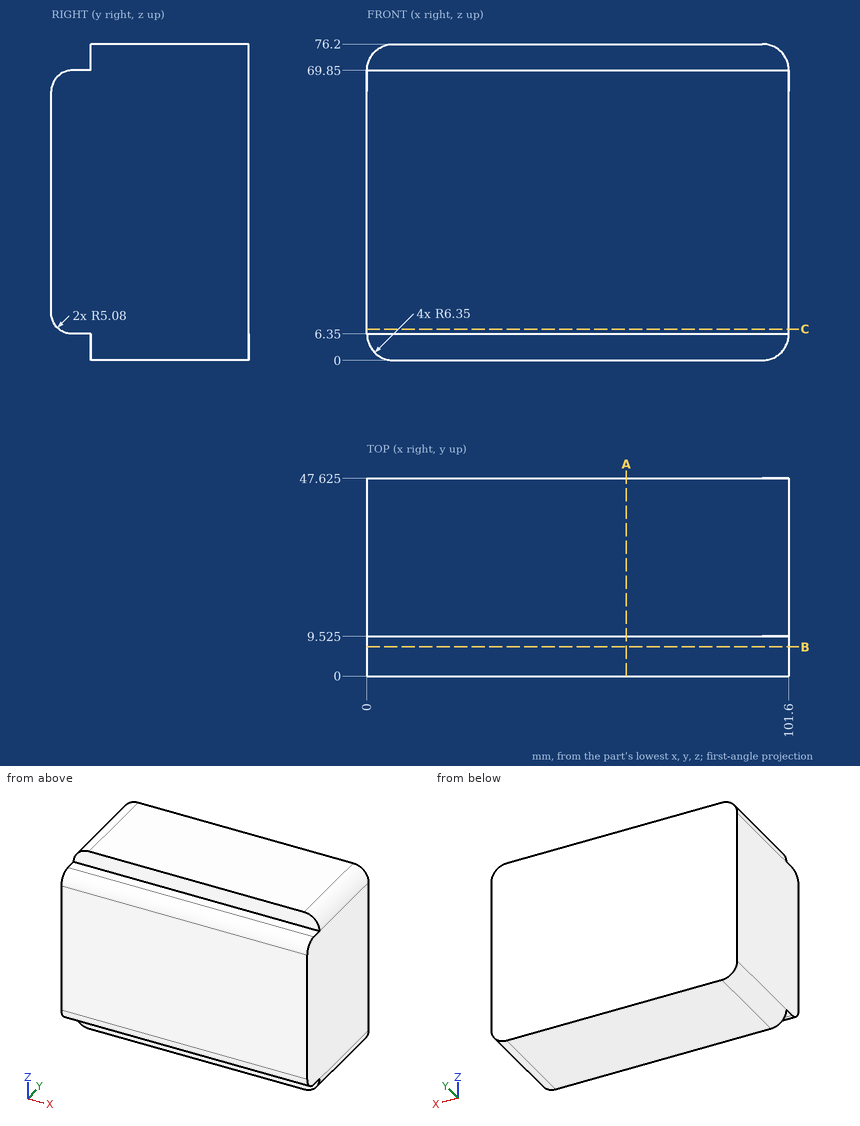
Geometry: see drawing. Coordinates: mm, zero at the bounding-box minimum. Round coordinates to 2 decimals unless told otherwise and drop trailing zeros. Loops run counter-clockwise (first coordinate to the right, second up) from the corner with the lowest first, then second, coordinate; pieces in that order, holes last. Notation, with made-up numbers: (84.25, 87.5) -> (125.25, 87.5) arc R28 cw to (125.25, 111.5) -> close; hole circle Ø10 at (-38, 24). An arc over 180 degrees is marked (long way). Write each question's results on one line, items separated by ' | '.
1. Section A-A (x = 62.5). Return loops of the section in (y, z) (3 decimals).
Geometry results:
outline: (0, 11.43) arc R5.08 ccw to (5.08, 6.35) -> (9.525, 6.35) -> (9.525, 0) -> (47.625, 0) -> (47.625, 76.2) -> (9.525, 76.2) -> (9.525, 69.85) -> (5.08, 69.85) arc R5.08 ccw to (0, 64.77) -> close
2. Section C-C (z = 7.5). Return loops of the section in (x, y) (3 decimals), and give its area (3 significant figures).
Geometry results:
outline: (0, 1.861) -> (101.6, 1.861) -> (101.6, 47.625) -> (0, 47.625) -> close | area: 4,650 mm2
3. First-contact query: P1, Ø5, axis at x = 74, z = 4.5, coming from the -Y side; P2, Ø1.9, axis at x = 73, z = 72.5, coming from the -Y side (3 decimals); P3, Ø1.3, axis at x = 27, y = 6.5, coming from the -Z side. Flat tips, straight axial feed; report the tip coordinate or a pass-through.
Geometry results:
P1: y = 2.59 | P2: y = 9.525 | P3: z = 6.35
4. Ray query, line 1 (X direction, y = 44, z = 6); line 2 (Y direction, x = 24, z = 70.5) (3 decimals); line 3 (Z direction, x = 46.5, y = 8). Return the intervals inside material, ascending. Write a range as from..to.
Geometry results:
line 1: 0.01..101.59 | line 2: 9.525..47.625 | line 3: 6.35..69.85
5. Section B-B (y = 7). Return loops of the section in (x, z).
Geometry results:
outline: (0, 6.35) -> (101.6, 6.35) -> (101.6, 69.85) -> (0, 69.85) -> close
